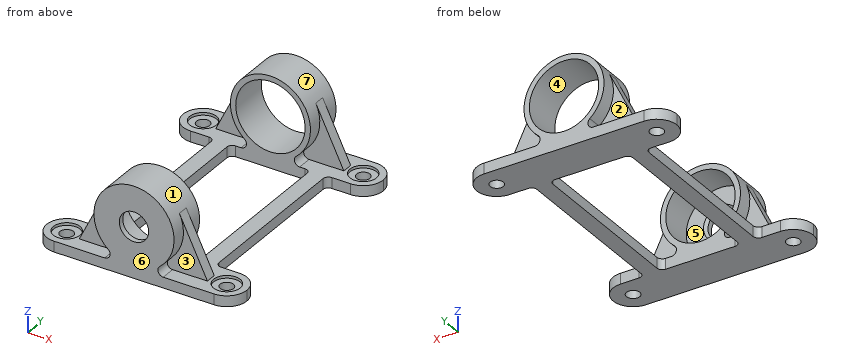
from build123d import *

# Parameters (mm, degrees)
F3_DEPTH       = 7.5
F4_R           = 7.49999
F6_D           = 5
F6_CBORE_D     = 10
F6_CBORE_DEPTH = 1
F8_DEPTH       = 2
F12_R          = 13
F13_DEPTH      = 92
F14_R          = 5.5
F15_DEPTH      = 95.001
F16_W          = 6
F16_H          = 4
F17_DEPTH      = 65
F18_R          = 2
F19_SIZE       = 1


# Not quite as in the source:
# - a fillet or chamfer is up to 0.001 mm smaller than in the source, because OpenCascade refuses the exact size


with BuildPart() as f3:
    # F2 (on Front) → F3 (new body, symmetric)
    with BuildSketch(Plane.XZ):
        with BuildLine():
            Line((-37.5, 0), (0, 0))
            Line((0, 0), (37.5, 0))
            Line((37.5, 0), (37.5, 4))
            Line((37.5, 4), (10.9544511501, 4))
            ThreePointArc((10.9544511501, 4), (9.0757782768, 5.3140056594), (9.6656921913, 7.5294117647))
            ThreePointArc((9.6656921913, 7.5294117647), (14.0900465494, 24.1449575543), (0, 34))
            ThreePointArc((0, 34), (-14.0900465494, 24.1449575543), (-9.6656921913, 7.5294117647))
            ThreePointArc((-9.6656921913, 7.5294117647), (-9.0757782768, 5.3140056594), (-10.9544511501, 4))
            Line((-10.9544511501, 4), (-37.5, 4))
            Line((-37.5, 4), (-37.5, 0))
        make_face()
    extrude(amount=F3_DEPTH, both=True)

    # F4 (radius 7.5 in the source; OpenCascade refuses exactly that, so slightly less here)
    f4_edges = [f3.edges().sort_by_distance(p)[0] for p in [
        (37.5, -7.5, 2),
        (37.5, 7.5, 2),
        (-37.5, -7.5, 2),
        (-37.5, 7.5, 2),
    ]]
    fillet(f4_edges, radius=F4_R)

    # F6 (through all)
    with Locations(Plane.XY.offset(4)):
        with Locations((30, 0), (-30, 0)):
            CounterBoreHole(F6_D / 2, F6_CBORE_D / 2, F6_CBORE_DEPTH)

    # F7 (on Front) → F8 (join, symmetric)
    with BuildSketch(Plane.XZ):
        with BuildLine():
            Line((10.9544511501, 4), (24, 4))
            Line((24, 4), (13.4831460674, 25.5730337079))
            ThreePointArc((13.4831460674, 25.5730337079), (14.6751576274, 15.8952055444), (9.6656921913, 7.5294117647))
            ThreePointArc((9.6656921913, 7.5294117647), (9.0757782768, 5.3140056594), (10.9544511501, 4))
        make_face()
    extrude(amount=F8_DEPTH, both=True)

    # F9: F3 across plane


with BuildPart() as f3_1:
    add(f3.part)
    add(f3.part.mirror(Plane.YZ))


with BuildPart() as f11_1:
    # F11: instance of F3
    add(f3_1.part.mirror(Plane.XZ.offset(40)))


with BuildPart() as f13_tool:
    # F12 (on face) → F13 (new body)
    with BuildSketch(Plane(origin=(0, 7.5, 0), x_dir=(-1, 0, 0), z_dir=(0, 1, 0))):
        with Locations((0, 19)):
            Circle(F12_R)
    extrude(amount=-F13_DEPTH)


with BuildPart() as f3_2:
    add(f3_1.part)

    # F13: cut by f13_tool
    add(f13_tool.part, mode=Mode.SUBTRACT)



with BuildPart() as f11_1_1:
    add(f11_1.part)

    # F13: cut by f13_tool
    add(f13_tool.part, mode=Mode.SUBTRACT)

    # F14 (on face) → F15 (cut, through all)
    with BuildSketch(Plane.XZ.offset(87.5)):
        with Locations((0, 19)):
            Circle(F14_R)
    extrude(amount=-F15_DEPTH, mode=Mode.SUBTRACT)


with BuildPart() as f3_3:
    add(f3_2.part)

    add(f11_1_1.part)  # F17 merges F11_1
    # F16 (on face) → F17 (join, through all)
    with BuildSketch(Plane.XZ.offset(7.5)):
        with Locations((18, 2)):
            Rectangle(F16_W, F16_H)
        with Locations((-18, 2)):
            Rectangle(F16_W, F16_H)
    extrude(amount=F17_DEPTH)

    # F18
    f18_edges = [f3_3.edges().sort_by_distance(p)[0] for p in [
        (21, -7.5, 2),
        (15, -7.5, 2),
        (21, -72.5, 2),
        (15, -72.5, 2),
        (-21, -7.5, 2),
        (-21, -72.5, 2),
        (-15, -72.5, 2),
        (-15, -7.5, 2),
    ]]
    fillet(f18_edges, radius=F18_R)

    # F19
    f19_edges = [f3_3.edges().sort_by_distance(p)[0] for p in [
        (-5.5, -84.5, 19),
    ]]
    chamfer(f19_edges, length=F19_SIZE)


solid = f3_3.part
Could you check a few things on this model? Use its own coordinates, in mm. Face numbers are marked on the shaded views. A direction names the side the tool comes from. Give positions to 0.01 mm unless a question says otherwise; leave off trailing zeros. Write each loop counter-clockwise with the first axis right and the second up, starting at its lowest first coordinate (ties: lowest second). Pieces come first, ordered by that corner, then holes. Notation, with made-up numbers: (-18.5, 85) -> (9.5, 85) arc R27 cw to (9.5, 123) -> close; hole circle Ø9 at (-17.75, 4.25). An arc over 180 degrees is marked (long way). Answer as a JSON object with one key per item and string values.
Q1. Please list where these lines run through material, in increasing order: L1, parallel to Y at x = 30, z = 2.1; L2, parallel to X at y = -33, z = 3; L3, parallel to Y at x = -8, z = 5.
Taken from the geometry:
{"L1": "y = -87.5 to -82.5, -77.5 to -72.5, -7.5 to -2.5, 2.5 to 7.5", "L2": "x = -21 to -15, 15 to 21", "L3": "y = -87.5 to -72.5, -7.5 to 7.5"}
Q2. Which directions (+Z, -Z, +X, -X, +Y, -Y) give clear straight access to the entire face, cutting with the end or side of a thin tool? Please do the marked faces 1, 2 and 3.
Taken from the geometry:
{"face 1": "none", "face 2": "-X, +Y", "face 3": "+X, -Y"}
Q3. Suppose I cut it at B-B on x = 0. Write out the boundary of the cut face in (y, z), then the cut area to 3 significant figures.
Taken from the geometry:
{"outline": "(-87.5, 0) -> (-72.5, 0) -> (-72.5, 6) -> (-84.5, 6) -> (-84.5, 12.5) -> (-85.5, 13.5) -> (-87.5, 13.5) -> close; (-87.5, 24.5) -> (-85.5, 24.5) -> (-84.5, 25.5) -> (-84.5, 32) -> (-72.5, 32) -> (-72.5, 34) -> (-87.5, 34) -> close; (-7.5, 0) -> (7.5, 0) -> (7.5, 6) -> (-7.5, 6) -> close; (-7.5, 32) -> (7.5, 32) -> (7.5, 34) -> (-7.5, 34) -> close", "area": "284 mm²"}
Q4. Will these pins go through, and if not, where does the flat tip stop? pin 1 Ø2 at (y, z) = (-47.5, 1.5) entering from -X; pin 2 Ø1.5 at (x, y) = (-23.5, -40.5) entering from -Z; pin 3 Ø15.5 at (x, z) = (0, 19) entering from +Y; pin 4 Ø12 at (x, z) = (-20, 12) entering from -Y.
Taken from the geometry:
{"pin 1": "stops at x = -21", "pin 2": "passes through", "pin 3": "stops at y = -84.5", "pin 4": "stops at y = -82"}
Q5. We'd pull the mould along X, two halves only. Please class the marked faces 4, 5, 6 and 7: released by +X, released by -X, zero draft, split by the parting line, or undercut.
Taken from the geometry:
{"face 4": "undercut", "face 5": "undercut", "face 6": "zero draft", "face 7": "split by the parting line"}
Q6. Suppose I cut it at C-C on z = 11. Count the separate pieces of the cut face and the enclosed holes in it, then the cut area to 3 significant figures.
Taken from the geometry:
{"separate pieces": "3", "enclosed holes": "0", "area": "334 mm²"}
Q7. Suppose I cut it at A-A on y = -19.5. Write out the boundary of the cut face in (x, z).
Taken from the geometry:
{"outline": "(-21, 0) -> (-15, 0) -> (-15, 4) -> (-21, 4) -> close; (15, 0) -> (21, 0) -> (21, 4) -> (15, 4) -> close"}
